Here's how the part is built. I have some questions about the finished solid (model axes, mm). A direction names the side the tool comes from. Round coordinates to 2 decimals unless told otherwise and drop trailing zeros. Write each loop counter-clockwise with the first axis right and the second up, starting at its lowest first coordinate (ties: lowest second). Pieces come first, ordered by that corner, then holes. Notation, with made-up numbers: (-16.5, -30.75) - (39.5, -30.75) arc R23 ccw to (39.5, -2.75) - close; hole circle Ø10 at (20.5, -4.75). An arc over 180 degrees is marked (long way). Use one line per item in the form item = value. Start each with the question number.
1. I want a section at B-B, the plane x = -147. List the corners of the cut face in (y, z) for me.
2. Will these pins go through, and if not, where does the flat tip stop? pin 1 (5 mm diameter, centred on y = -11.5, z = -266.5, fed in from -X); pin 2 (6 mm diameter, centred on x = -18, z = -237.5, fed in from +Y); pin 3 (8.5 mm diameter, centred on x = -118, y = -9.5, fed in from +Z).
3. If I drill on line 1 along Z through (x, y) = (-105, -3.25); line 2 along X through (y, z) = (-11.75, -322); line 3 along X through (y, z) = (-9.5, -427), over which ranges is the centre line in solid material (lowest first)?
4. I want a section at C-C, the plane z = -205.5. List the corners of the cut face in (x, y) for me.
5. I want a section at A-A, the plane y = -12.75. List the corners of the cut face in (x, z) for me, plus the area to 3 significant figures.
6. Which directions (+Z, -Z, +X, -X, +Y, -Y) give clear straight access to the entire face, cutting with the end or side of a thin tool? Please do faces 1 (the flat face through (-0.055, -8, -276)), 2 (the flat face through (-25.455, -8, -131)), 3 (the flat face through (-95.305, -8, -131)).
```python
from build123d import *

# Parameters (mm, degrees)
F1_DEPTH = 16.51
F2_R     = 38.1
F3_R     = 38.1


with BuildPart() as f1:
    # F0 (on Front) → F1 (new body)
    with BuildSketch(Plane.XZ):
        Polygon((-0.055255, -445.639101), (-0.055255, -140.839101), (-25.455255, -140.839101), (-25.455255, -121.789101), (-95.305255, -121.789101), (-95.305255, -140.839101), (-127.055255, -140.827884), (-177.855255, -445.639101), align=None)
    extrude(amount=F1_DEPTH)

    # F2
    f2_edges = [f1.edges().sort_by_distance(p)[0] for p in [
        (-177.855255, -8.255, -445.639101),
    ]]
    fillet(f2_edges, radius=F2_R)

    # F3
    f3_edges = [f1.edges().sort_by_distance(p)[0] for p in [
        (-0.055255, -8.255, -445.639101),
    ]]
    fillet(f3_edges, radius=F3_R)


solid = f1.part
```
Model answer:
q1.outline = (-16.51, -442.93) - (0, -442.93) - (0, -260.5) - (-16.51, -260.5) - close
q2.pin_1 = -148.42
q2.pin_2 = 0
q2.pin_3 = -140.83
q3.line_1 = -445.64 to -140.84
q3.line_2 = -157.25 to -0.06
q3.line_3 = -165.63 to -5.4
q4.outline = (-137.83, -16.51) - (-0.06, -16.51) - (-0.06, 0) - (-137.83, 0) - close
q5.outline = (-170.46, -401.28) arc R38.1 ccw to (-132.88, -445.64) - (-38.16, -445.64) arc R38.1 ccw to (-0.06, -407.54) - (-0.06, -140.84) - (-25.46, -140.84) - (-25.46, -121.79) - (-95.31, -121.79) - (-95.31, -140.84) - (-127.06, -140.83) - close
q5.area = 47,000 mm2
q6.face_1 = +Z, -Z, +X, +Y, -Y
q6.face_2 = +Z, +X, +Y, -Y
q6.face_3 = +Z, -X, +Y, -Y
